For this review, take the finished solid that the model builds, in its own axes (mm). Face numbers are marked on the shaded views. A direction names the side the tool comes from. Coordinates: 2 decimals unless noted, no trailing zeros. Loops run counter-clockwise (first coordinate to the right, second up) from the corner with the lowest first, then second, coordinate; pieces in that order, holes last. Notation, with made-up numbers: M 14.5,18.5 L 53.5,18.5 A20 cw 53.5,37.5 Z; hole C 26,-2 d11. An arc over 180 degrees is marked long. Write item = value, one per line.
from build123d import *

# Parameters (mm, degrees)
F0_W     = 139.7
F0_H     = 139.7
F1_DEPTH = 6.35
F2_W     = 101.6
F2_H     = 101.6
F3_DEPTH = 6.35
F4_R     = 5.08


with BuildPart() as f1:
    # F0 (on Top) → F1 (new body)
    with BuildSketch(Plane.XY):
        Rectangle(F0_W, F0_H)
    extrude(amount=F1_DEPTH)

    # F2 (on face) → F3 (join)
    with BuildSketch(Plane.XY.offset(6.35)):
        Rectangle(F2_W, F2_H)
    extrude(amount=F3_DEPTH)

    # F4
    f4_edges = [f1.edges().sort_by_distance(p)[0] for p in [
        (50.8, -50.8, 9.525),
        (50.8, 50.8, 9.525),
        (-50.8, -50.8, 9.525),
        (-50.8, 50.8, 9.525),
    ]]
    fillet(f4_edges, radius=F4_R)


solid = f1.part
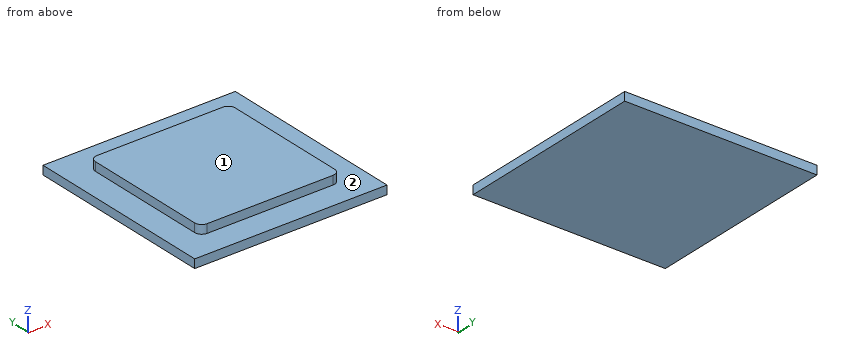
Q1. For pin 1 Ø7 at (x, z) = (-19, 10.5) entering from -Y; pin 2 Ø1.9 at (y, z) = (-4, 10.5) entering from +X; pin 3 Ø5 at (y, z) = (15, 9) entering from -X, all flat-tipped, find the tip position at first contact; note any pin that passes through.
Solved:
pin_1 = -50.8
pin_2 = 50.8
pin_3 = -50.8
Q2. Add section B-B (z = 8). Write out the cut boundary in (x, y), and give its area (3 significant figures).
Solved:
outline = M -50.8,-45.72 A5.08 ccw -45.72,-50.8 L 45.72,-50.8 A5.08 ccw 50.8,-45.72 L 50.8,45.72 A5.08 ccw 45.72,50.8 L -45.72,50.8 A5.08 ccw -50.8,45.72 Z
area = 10,300 mm²
Q3. Add section A-A (y = -17). Write out the cut boundary in (x, z), and give its area (3 significant figures).
Solved:
outline = M -69.85,0 L 69.85,0 L 69.85,6.35 L 50.8,6.35 L 50.8,12.7 L -50.8,12.7 L -50.8,6.35 L -69.85,6.35 Z
area = 1,530 mm²
Q4. Machinability: for the marked faces 1 and 2, which of the approach directions +Z, -Z, +X, -X, +Y, -Y give a long, thin tool a straight path to every point of the face, cutting with its end or side? Answer none if there is none.
Solved:
face_1 = +Z, +X, -X, +Y, -Y
face_2 = +Z
Q5. For line 1 along Z through (x, y) = (61, -62); line 2 along Y through (x, z) = (36.5, 9.5), list the stretches that pass through material, from the lowest coordinate up.
Solved:
line_1 = 0 to 6.35
line_2 = -50.8 to 50.8
Q6. Add section C-C (x = -60). Write out the cut boundary in (y, z), and give its area (3 significant figures).
Solved:
outline = M -69.85,0 L 69.85,0 L 69.85,6.35 L -69.85,6.35 Z
area = 887 mm²
